Read the model definition and answer for the solid it produces. Units are mm, in the model's axes. A direction names the side the tool comes from. Coordinates: 2 decimals unless noted, no trailing zeros. Write each loop counter-clockwise with the first axis right and the second up, starting at its lowest first coordinate (ties: lowest second). Pieces come first, ordered by that corner, then holes. Notation, with made-up numbers: (8.25, 47.5) - (30.25, 47.5) arc R27 cw to (30.25, 66.5) - close; hole circle Ø4 at (-3, -39.5). An arc over 180 degrees is marked (long way). Use a Markdown table: item, result.
from build123d import *

# Parameters (mm, degrees)
SKETCH2_W            = 72.4
SKETCH2_H            = 24
BOSS_EXTRUDE3_DEPTH  = 24
SKETCH5_W            = 24
SKETCH5_H            = 24
BOSS_EXTRUDE4_DEPTH  = 72.4
SKETCH6_R            = 1.7
CUT_EXTRUDE2_DEPTH   = 111.505746457
LPATTERN1_COUNT      = 2
LPATTERN1_PITCH      = 8
LPATTERN1_COUNT_DIR2 = 2
LPATTERN1_PITCH_DIR2 = 24.13
SKETCH7_R            = 11.5
CUT_EXTRUDE3_DEPTH   = 4
SKETCH8_R            = 9.5
CUT_EXTRUDE4_DEPTH   = 2
SKETCH9_R            = 3
CUT_EXTRUDE5_DEPTH   = 7


with BuildPart() as part:
    # Sketch2 → Boss-Extrude3 (new body)
    with BuildSketch(Plane(origin=(0, 0, 0), x_dir=(0, 0, -1), z_dir=(1, 0, 0))):
        with Locations((-36.2, 12)):
            Rectangle(SKETCH2_W, SKETCH2_H)
    extrude(amount=BOSS_EXTRUDE3_DEPTH)

    # Sketch5 → Boss-Extrude4 (add)
    with BuildSketch(Plane(origin=(0, 24, 0), x_dir=(1, 0, 0), z_dir=(0, 1, 0))):
        with Locations((12, -12)):
            Rectangle(SKETCH5_W, SKETCH5_H)
    extrude(amount=BOSS_EXTRUDE4_DEPTH)

    # Sketch6 → Cut-Extrude2 (cut, symmetric)
    with BuildSketch(Plane.XY.offset(24)):
        with Locations((8, 72.266666667)):
            Circle(SKETCH6_R)
    cut_extrude2 = extrude(amount=CUT_EXTRUDE2_DEPTH, both=True, mode=Mode.SUBTRACT)

    # LPattern1: Cut-Extrude2 2 × 2
    with Locations(*[(i * LPATTERN1_PITCH, -j * LPATTERN1_PITCH_DIR2, 0) for i in range(LPATTERN1_COUNT) for j in range(LPATTERN1_COUNT_DIR2) if (i, j) != (0, 0)]):
        add(cut_extrude2, mode=Mode.SUBTRACT)

    # Sketch7 → Cut-Extrude3 (cut)
    with BuildSketch(Plane(origin=(0, 24, 0), x_dir=(1, 0, 0), z_dir=(0, 1, 0))):
        with Locations(Location((12, -36.2, 0), (0, 0, 270))):
            Circle(SKETCH7_R)
    extrude(amount=-CUT_EXTRUDE3_DEPTH, mode=Mode.SUBTRACT)

    # Sketch8 → Cut-Extrude4 (cut)
    with BuildSketch(Plane(origin=(0, 20, 0), x_dir=(1, 0, 0), z_dir=(0, 1, 0))):
        with Locations(Location((12, -36.2, 0), (0, 0, 270))):
            Circle(SKETCH8_R)
    extrude(amount=-CUT_EXTRUDE4_DEPTH, mode=Mode.SUBTRACT)

    # Sketch9 → Cut-Extrude5 (cut)
    with BuildSketch(Plane(origin=(0, 18, 0), x_dir=(1, 0, 0), z_dir=(0, 1, 0))):
        with Locations(Location((12, -36.2, 0), (0, 0, 270))):
            Circle(SKETCH9_R)
    extrude(amount=-CUT_EXTRUDE5_DEPTH, mode=Mode.SUBTRACT)


solid = part.part
(1) For faces 1 (the cylindrical face through (7.779, 49.822, 12.168)), 2 (the flat face through (14.24, 18, 33.96)), 3 (the flat face through (12, 60, 24)), determine the directions among +Z, -Z, +X, -X, +Y, -Y from which every point of the face is accessible in a straight line to the end or side of a thin tool.
Report:
| item | result |
|---|---|
| face 1 | +Z, -Z |
| face 2 | +Y |
| face 3 | +Z, +X, -X, +Y |
(2) A cutting plane is placed at D-D, the plane y = 37.5. Write down the section's boundary in (x, z).
Report:
| item | result |
|---|---|
| outline | (0, 0) - (24, 0) - (24, 24) - (0, 24) - close |
(3) Each of these flat-tipped pins is pushed along its axis until it touches: P1, Ø11.5, axis at x = 12, z = 36.2, coming from the +Y side; P2, Ø6, axis at x = 21, z = 36, coming from the +Y side; P3, Ø7, axis at x = 10.5, y = 66, coming from the +Z side. Where does it stop, or does it pass through?
Report:
| item | result |
|---|---|
| P1 | stops at y = 18 |
| P2 | stops at y = 24 |
| P3 | stops at z = 24 |
(4) The mould has two halves that part along X. Classify faces 4 (the flat face through (12, 12, 72.4)), 5 (the cylindrical face through (15.779, 49.822, 12.168)), 6 (the flat face through (0, 37, 21)): pulls with the +X half, pulls with the -X half, needs draft (parallel to the pull), parting line crosses it, or undercut.
Report:
| item | result |
|---|---|
| face 4 | needs draft |
| face 5 | undercut |
| face 6 | pulls with the -X half |
(5) A cutting plane is placed at C-C, the plane z = 36.2. Write down the section's boundary in (x, y), and give its area (3 significant figures).
Report:
| item | result |
|---|---|
| outline | (0, 0) - (24, 0) - (24, 24) - (23.5, 24) - (23.5, 20) - (21.5, 20) - (21.5, 18) - (15, 18) - (15, 11) - (9, 11) - (9, 18) - (2.5, 18) - (2.5, 20) - (0.5, 20) - (0.5, 24) - (0, 24) - close |
| area | 404 mm² |
(6) Straight lines are drawn through the part: L1, parallel to Y at x = 8, z = 9.25; L2, parallel to X at y = 15.25, z = 36.2; L3, parallel to Y at x = 3, z = 66. For each, find the intervals that lie inside material, in ascending order.
Report:
| item | result |
|---|---|
| L1 | y = 0 to 46.44, 49.84 to 70.57, 73.97 to 96.4 |
| L2 | x = 0 to 9, 15 to 24 |
| L3 | y = 0 to 24 |
(7) A cutting plane is placed at B-B, the plane z = 12. Write down the section's boundary in (x, y), and give its area (3 significant figures).
Report:
| item | result |
|---|---|
| outline | (0, 0) - (24, 0) - (24, 96.4) - (0, 96.4) - close; hole circle Ø3.4 at (8, 48.14); hole circle Ø3.4 at (8, 72.27); hole circle Ø3.4 at (16, 48.14); hole circle Ø3.4 at (16, 72.27) |
| area | 2,280 mm² |
(8) A cutting plane is placed at A-A, the plane x = 16. Write down the section's boundary in (y, z).
Report:
| item | result |
|---|---|
| outline | (0, 0) - (46.44, 0) - (46.44, 24) - (24, 24) - (24, 25.42) - (20, 25.42) - (20, 27.58) - (18, 27.58) - (18, 44.82) - (20, 44.82) - (20, 46.98) - (24, 46.98) - (24, 72.4) - (0, 72.4) - close; (49.84, 0) - (70.57, 0) - (70.57, 24) - (49.84, 24) - close; (73.97, 0) - (96.4, 0) - (96.4, 24) - (73.97, 24) - close |
